from build123d import *

# Parameters (mm, degrees)
F0_W     = 64
F0_H     = 104
F1_DEPTH = 5
F2_W     = 5
F2_H     = 20
F3_DEPTH = 25
F5_W     = 8
F5_H     = 25
F6_DEPTH = 25
F8_DEPTH = 25


with BuildPart() as f1:
    # F0 (on Top) → F1 (new body)
    with BuildSketch(Plane.XY):
        Rectangle(F0_W, F0_H)
    extrude(amount=F1_DEPTH)

    # F2 (on face) → F3 (cut)
    with BuildSketch(Plane.XY.offset(5)):
        with Locations((29.5, 0)):
            Rectangle(F2_W, F2_H)
    extrude(amount=-F3_DEPTH, mode=Mode.SUBTRACT)

    # F5 (on face) → F6 (cut)
    with BuildSketch(Plane.XY.offset(5)):
        with Locations((0, 27.5)):
            Rectangle(F5_W, F5_H)
    extrude(amount=-F6_DEPTH, mode=Mode.SUBTRACT)

    # F7 (on face) → F8 (join)
    with BuildSketch(Plane(origin=(4, 0, 0), x_dir=(0, -1, 0), z_dir=(-1, 0, 0))):
        with BuildLine():
            Line((-15, 5), (-35, 5))
            add(Edge.make_bspline(
                [(-35, 5), (-27.9895598193, 1.8046537073), (-18.7225920955, 0.0081415234), (-15, 0)],
                knots=[0, 0, 0, 0, 20.6155281281, 20.6155281281, 20.6155281281, 20.6155281281], degree=3))
            Line((-15, 0), (-15, 5))
        make_face()
    extrude(amount=F8_DEPTH)


solid = f1.part
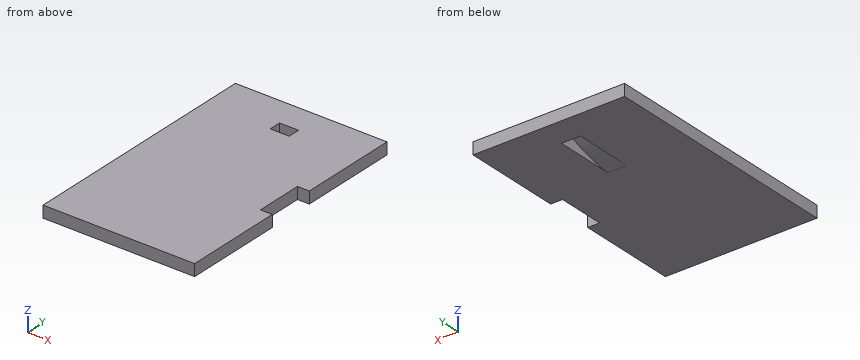
The model under review builds one solid part; all positions refer to its coordinate system, in mm. Give positions to 0.01 mm unless a question says otherwise; leave off trailing zeros. Write each loop counter-clockwise with the first axis right and the second up, starting at its lowest first coordinate (ties: lowest second). Pieces come first, ordered by that corner, then holes. Notation, with made-up numbers: M 76,6.25 L 116,6.25 A13 ccw 116,12.25 Z; hole C 73,21.5 d10. An arc over 180 degrees is marked long. One line per question, with ' | ' between items. Start each with the question number.
Item 1: We need section A-A on y = 4. Write out the cut boundary in (x, z), plus the area to 3 significant figures.
Item 2: Wall thickness on line 1 (X direction, y = 29, z = 1.3); line 2 (X direction, y = -8, z = 2.1): over which ranges is each line inside the solid? List them lowest first. Write a range as from..to.
Item 3: For pin 1 (3 mm diameter, centred on x = 6, y = -5.5, fed in from -Z); pin 2 (1.5 mm diameter, centred on y = -4, z = 2.5, fed in from +X), all flat-tipped, find the tip position at first contact; note any pin that passes through.
Results found:
1) outline: M -32,0 L 27,0 L 27,5 L -32,5 Z | area: 295 mm2
2) line 1: x = -32..-4, 4..32 | line 2: x = -32..27
3) pin 1: stops at z = 0 | pin 2: stops at x = 27
